Check sheet for the modelled part. Datum: model origin and axes. Units: mm. A direction names the side the tool comes from. Coordinates: 2 decimals unless noted, no trailing zeros. Loops run counter-clockwise (first coordinate to the right, second up) from the corner with the lowest first, then second, coordinate; pieces in that order, holes last. Notation, with made-up numbers: (0.5, 1.5) - (53.5, 1.5) arc R26 cw to (53.5, 40.5) - close; hole circle Ø9 at (21, 58). An arc over 180 degrees is marked (long way). Write each question's results on one line, items separated by ' | '. Start each with the question number.
1. Gauge pin test, flat ends, axial feed: P1, Ø9, axis at y = -1.5, z = 32.5, coming from the +X side; P2, Ø1.5, axis at y = 0.5, z = -26.5, coming from the -X side; P3, Ø1, axis at y = 6.5, z = -35, coming from the +X side. Record the tip position at first contact, or that the pin passes through.
2. Cross-section at A-A (y = 0). Record the cut outline in (x, z).
3. Draft check along X on faces 1 (the face through (-26, 0, 22)), 2 (the face through (-2.17, -9.76, -15.14)), 3 (the face through (-1.73, -7.81, -17.11)), 4 (the face through (-24.06, 3, 39.54)). Enter one of: released by +X, released by -X, zero draft, split by the parting line, or undercut.
4. Cross-section at C-C (x = -25.5). Record the cut outline in (y, z), and give its area (3 significant figures).
5. Cross-section at D-D (y = -11.5). Record the cut outline in (x, z).
6. Cross-section at B-B (z = 5). Record the cut outline in (x, y).
7. Thickness scan on line 1 (Z direction, x = -27.25, y = 0); line 2 (X direction, y = 3.75, z = 17.5); line 3 (Y direction, x = -25.75, z = 30). Record the ranges inside material, lowest first. Write a range as [from, to].
8. Tool access check on faces 5 (the face through (-28, 10, 27)), 6 (the face through (-29.014, -11.056, 40.138)). Record the directions out of +Z, -Z, +X, -X, +Y, -Y that give a thin tool (end or side, any length) a straight path to the whole face; none if there is none.
```python
from build123d import *

# Parameters (mm, degrees)
F2_R     = 10
F2_R_2   = 8
F7_R     = 15
F7_R_2   = 10
F8_DEPTH = 2


# Not quite as in the source:
# - a fillet or chamfer that OpenCascade refuses, or shapes differently, is made with other operations: its cross-section is extruded or revolved along the edge and cut away or added


with BuildPart() as f3:
    # F3: sweep along a path in F0
    with BuildLine(Plane.XZ) as f3_path:
        Line((0, -45), (0, 10))
        ThreePointArc((0, 10), (-5.8578643763, 24.1421356237), (-20, 30))
        Line((-20, 30), (-35, 30))
    # F2 (on plane+point) → F3 (sweep)
    with BuildSketch(Plane.XY.offset(-45)):
        Circle(F2_R)
        Circle(F2_R_2, mode=Mode.SUBTRACT)
    sweep(path=f3_path.line)

    # F4: fillet of radius 5 on 1 edges, made by hand

    # F4_s1 → F4_t2 (revolve, cut)
    with BuildSketch(Plane.XZ):
        with BuildLine():
            ThreePointArc((10, -41), (9.472135955, -43.2360679775), (8, -45))
            Line((8, -45), (10, -45))
            Line((10, -45), (10, -41))
        make_face()
    revolve(axis=Axis((0, 0, -45), (0, 0, 1)), mode=Mode.SUBTRACT)

    # F5: fillet of radius 5 on 1 edges, made by hand

    # F5_s1 → F5_t2 (revolve, cut)
    with BuildSketch(Plane.XZ):
        with BuildLine():
            ThreePointArc((-35, 40), (-33.2360679775, 38.527864045), (-31, 38))
            Line((-31, 38), (-35, 38))
            Line((-35, 38), (-35, 40))
        make_face()
    revolve(axis=Axis((-35, 0, 30), (-1, 0, 0)), mode=Mode.SUBTRACT)

    # F7 (on offset) → F8 (join)
    with BuildSketch(Plane.YZ.offset(-30)):
        with Locations((0, 30)):
            Circle(F7_R)
        with Locations((0, 30)):
            Circle(F7_R_2, mode=Mode.SUBTRACT)
    extrude(amount=F8_DEPTH)


solid = f3.part
```
Established:
1) P1: x = 3.92 | P2: x = -10 | P3: x = 8
2) outline: (-35, 20) - (-30, 20) - (-30, 15) - (-28, 15) - (-28, 20) - (-20, 20) arc R10 cw to (-10, 10) - (-10, -41) arc R5 ccw to (-8, -45) - (-8, 10) arc R12 ccw to (-20, 22) - (-31, 22) arc R5 ccw to start; (-35, 40) arc R5 ccw to (-31, 38) - (-20, 38) arc R28 cw to (8, 10) - (8, -45) arc R5 ccw to (10, -41) - (10, 10) arc R30 ccw to (-20, 40) - (-28, 40) - (-28, 45) - (-30, 45) - (-30, 40) - close
3) face 1: zero draft | face 2: split by the parting line | face 3: undercut | face 4: undercut
4) outline: circle Ø20 at (0, 30); hole circle Ø16 at (0, 30) | area: 113 mm^2
5) outline: (-30, 20.37) - (-28, 20.37) - (-28, 39.63) - (-30, 39.63) - close
6) outline: circle Ø20 at (0, 0); hole circle Ø16 at (0, 0)
7) line 1: [20, 22], [38, 40] | line 2: [-30, -28], [-12.33, -9.46], [6.01, 8.29] | line 3: [-10, -8], [8, 10]
8) face 5: none | face 6: -X
